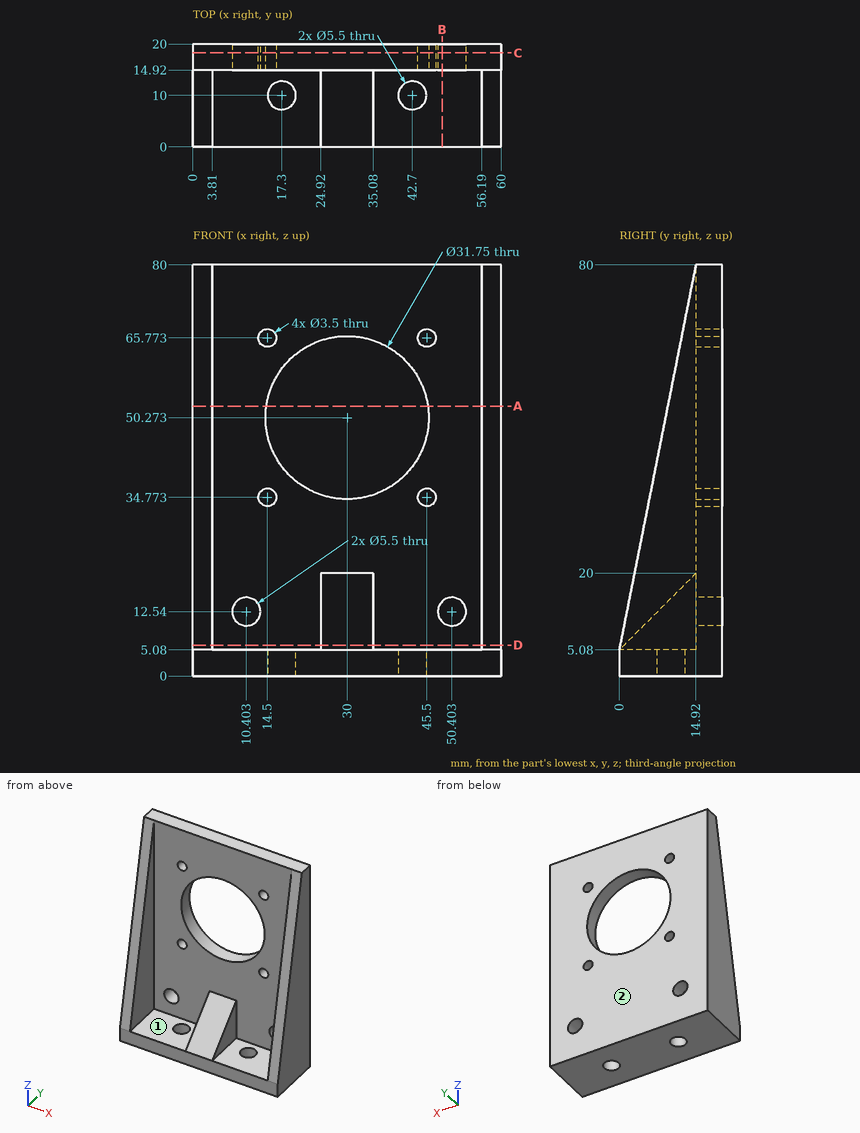
Geometry: see drawing. Coordinates: mm, zero at the bounding-box minimum. A direction names the side the tool comes from. Coordinates: 2 decimals unless noted, no trailing zeros. Write each loop counter-clockwise with the first axis right and the second up, starting at its lowest first coordinate (ties: lowest second). Pieces come first, ordered by that corner, then holes. Notation, with made-up numbers: (-17.75, 39.25) - (33.25, 39.25) arc R22 ccw to (33.25, 49.25) - close; hole circle Ø4 at (34.5, -4.5). An arc over 180 degrees is marked (long way). Put each result on its own line as item: value. Start each with the question number.
1) Ray query, L1, parallel to Y at x = 17.3, z = 1.5; L2, parallel to Z at x = 30, y = 16.9; L3, parallel to X at y = 13.5, z = 64. Return the intervals inside material, ascending.
2) Cut plane B-B (x = 48.5). Return the cut outline in (y, z) (1 decimal).
3) Cut plane C-C (y = 18.25). State how many separate pieces and enclosed holes the cut face has, plus the area to 3 significant figures.
4) Cut plane D-D (z = 6). Return the cut outline in (x, y).
5) Cut plane A-A (z = 52.5). Return the cut outline in (x, y).
6) Reachability of the marked faces 1 and 2 from +Z, -Z, +X, -X, +Y, -Y: full face, straight path, thin tool, end or side. Return the list, or none.
7) Contact query for flat-ended pins moving along their axis: pin 1 (12 mm diameter, centred on x = 44.5, y = 8, fed in from +Z); pin 2 (3.5 mm diameter, centred on x = 42.7, y = 10, fed in from -Z); pin 3 (15.5 mm diameter, centred on x = 21.5, z = 52, fed in from -Y); pin 4 (12 mm diameter, centred on x = 24.5, y = 8.5, fed in from +Z) (1 decimal). Output: stop coordinate, or through.
Resolved:
1. L1: y = 0 to 7.25, 12.75 to 20
1. L2: z = 0 to 34.4, 66.15 to 80
1. L3: x = 0 to 3.81, 56.19 to 60
2. outline: (0, 0) - (20, 0) - (20, 10.6) - (14.9, 10.6) - (14.9, 5.1) - (0, 5.1) - close; (14.9, 14.5) - (20, 14.5) - (20, 80) - (14.9, 80) - close
3. separate pieces: 1
3. enclosed holes: 7
3. area: 3,920 mm2
4. outline: (0, 0.18) - (3.81, 0.18) - (3.81, 14.92) - (24.92, 14.92) - (24.92, 0.92) - (35.08, 0.92) - (35.08, 14.92) - (56.19, 14.92) - (56.19, 0.18) - (60, 0.18) - (60, 20) - (0, 20) - close
5. outline: (0, 9.44) - (3.81, 9.44) - (3.81, 14.92) - (14.28, 14.92) - (14.28, 20) - (0, 20) - close; (45.72, 14.92) - (56.19, 14.92) - (56.19, 9.44) - (60, 9.44) - (60, 20) - (45.72, 20) - close
6. face 1: +Z, -Y
6. face 2: +Z, -Z, +X, -X, +Y
7. pin 1: stops at z = 5.08
7. pin 2: passes through
7. pin 3: stops at y = 14.92
7. pin 4: stops at z = 19.6
